Part model, mm, in its own coordinate system. Face numbers are marked on the shaded views. A direction names the side the tool comes from. Round coordinates to 2 decimals unless told otherwise and drop trailing zeros. Order: outer loops, then holes, each group sorted by start corner. A loop starts at its lowest first (then second) coordinate and runs counter-clockwise, first axis right, second up. Notation, with made-up numbers: M 43.25,-29.75 L 51.25,-29.75 A26 ccw 51.25,-3.75 Z; hole C 5.5,40 d2. An arc over 180 degrees is marked long. One line per question, with ' | ' between items.
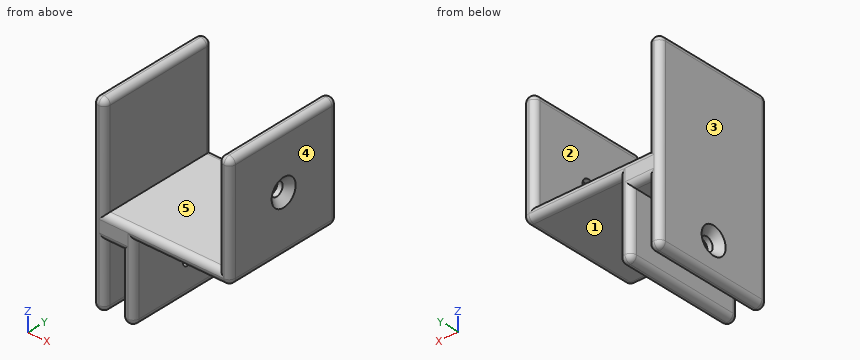
from build123d import *

# Parameters (mm, degrees)
F1_DEPTH       = 30
F3_D           = 3.3
F3_DEPTH       = 13.5
F3_CSINK_D     = 6.72
F3_CSINK_ANGLE = 90
F3_TIP         = 0.9914200214
F4_R           = 1.49999
F6_D           = 3.3
F6_DEPTH       = 7
F6_CSINK_D     = 6.72
F6_CSINK_ANGLE = 90
F6_TIP         = 0.9914200214
F8_D           = 2.5
F8_DEPTH       = 7
F8_TIP         = 0.7510757738


# Not quite as in the source:
# - a fillet or chamfer is up to 0.001 mm smaller than in the source, because OpenCascade refuses the exact size


with BuildPart() as f1:
    # F0 (on Front) → F1 (new body)
    with BuildSketch(Plane.XZ):
        Polygon((0, 28), (0, 0), (0, -19), (3, -19), (3, -3), (7.2, -3), (7.2, -19), (10.2, -19), (10.2, 0), (34.1, 0), (34.1, 28), (31.1, 28), (31.1, 3), (3, 3), (3, 28), align=None)
    extrude(amount=F1_DEPTH)

    # F3
    with Locations(Plane.YZ.offset(34.1)):
        with Locations((-15, 14)):
            CounterSinkHole(F3_D / 2, F3_CSINK_D / 2, depth=F3_DEPTH, counter_sink_angle=F3_CSINK_ANGLE)
            with Locations((0, 0, -(F3_DEPTH + F3_TIP / 2))):  # 118° drill point
                Cone(0, F3_D / 2, F3_TIP, mode=Mode.SUBTRACT)

    # F4 (radius 1.5 in the source; OpenCascade refuses exactly that, so slightly less here)
    f4_edges = [f1.edges().sort_by_distance(p)[0] for p in [
        (0, -15, -19),
        (3, -15, -19),
        (7.2, -15, -19),
        (10.2, -15, -19),
        (31.1, -15, 28),
        (34.1, -15, 28),
        (3, -15, 28),
        (0, -15, 28),
        (1.5, -30, 28),
        (32.6, -30, 28),
        (31.1, -30, 15.5),
        (34.1, -30, 14),
        (3, -30, 15.5),
        (0, -30, 4.5),
        (17.05, -30, 3),
        (22.15, -30, 0),
        (10.2, -30, -9.5),
        (1.5, -30, -19),
        (8.7, -30, -19),
        (1.5, 0, -19),
        (8.7, 0, -19),
        (0, 0, 4.5),
        (3, 0, -11),
        (7.2, 0, -11),
        (10.2, 0, -9.5),
        (17.05, 0, 3),
        (3, 0, 15.5),
        (22.15, 0, 0),
        (34.1, 0, 14),
        (34.1, -15, 0),
        (5.1, 0, -3),
        (5.1, -30, -3),
        (32.6, 0, 28),
        (1.5, 0, 28),
        (31.1, 0, 15.5),
        (3, -30, -11),
        (7.2, -30, -11),
    ]]
    fillet(f4_edges, radius=F4_R)

    # F6
    with Locations(Plane(origin=(0, 0, 0), x_dir=(0, -1, 0), z_dir=(-1, 0, 0))):
        with Locations((15, -11)):
            CounterSinkHole(F6_D / 2, F6_CSINK_D / 2, depth=F6_DEPTH, counter_sink_angle=F6_CSINK_ANGLE)
            with Locations((0, 0, -(F6_DEPTH + F6_TIP / 2))):  # 118° drill point
                Cone(0, F6_D / 2, F6_TIP, mode=Mode.SUBTRACT)

    # F8
    with Locations(Plane.YZ.offset(10.2)):
        with Locations((-15, -11)):
            Hole(F8_D / 2, depth=F8_DEPTH)
            with Locations((0, 0, -(F8_DEPTH + F8_TIP / 2))):  # 118° drill point
                Cone(0, F8_D / 2, F8_TIP, mode=Mode.SUBTRACT)


solid = f1.part
1) Drop flat-ended pins along their axis: pin 1 (11 mm diameter, centred on x = 20, y = -21, fed in from -Z); pin 2 (5.5 mm diameter, centred on y = -14, z = -6.5, fed in from +X); pin 3 (3 mm diameter, centred on y = -15, z = -11, fed in from -X). Give the stop position or say it passes through.
The answers:
pin 1: stops at z = 0 | pin 2: stops at x = 10.2 | pin 3: stops at x = 7.2
2) Saw through at B-B (x = 4.5). List the corners of the cut face in (y, z).
The answers:
outline: M -30,-1.5 A1.5 ccw -28.5,-3 L -1.5,-3 A1.5 ccw 0,-1.5 L 0,1.5 A1.5 ccw -1.5,3 L -28.5,3 A1.5 ccw -30,1.5 Z
3) Probe line 1 (X direction, y = -6.75, z = 5.5); line 2 (X direction, y = -20, z = -7); line 3 (Z direction, x = 30, y = -25.25). List the from-to ranges inside material, lowest first. Write a range as [from, to].
The answers:
line 1: x = [0, 3], [31.1, 34.1] | line 2: x = [0, 3], [7.2, 10.2] | line 3: z = [0, 3]
4) Saw through at A-A (z = -11). Give the number of separate pieces and of enclosed holes in the cut face, plus the area to 3 significant figures.
The answers:
separate pieces: 4 | enclosed holes: 0 | area: 156 mm²
5) Two-plate mould, pull along X, no slides. Class the marked faces 3, 4 and 5: released by +X, released by -X, zero draft, split by the parting line, or undercut.
The answers:
face 3: released by -X | face 4: released by +X | face 5: undercut
6) Which spindle directions (+Z, -Z, +X, -X, +Y, -Y) get a long thin tool onto all of the face, cutting with end or side? Do the marked faces 1 and 2. Say none if no direction does.
The answers:
face 1: -Z, +X, +Y, -Y | face 2: +Z, +Y, -Y
